from build123d import *

# Parameters (mm, degrees)
CROQUIS1_W              = 32
CROQUIS1_H              = 74.5
CROQUIS1_R              = 1.5
SALIENTE_EXTRUIR1_DEPTH = 1.5
REDONDEO1_R             = 2


with BuildPart() as part:
    # Croquis1 → Saliente-Extruir1 (new, symmetric)
    with BuildSketch(Plane.XY):
        Rectangle(CROQUIS1_W, CROQUIS1_H)
        with Locations((0, 27.25)):
            Circle(CROQUIS1_R, mode=Mode.SUBTRACT)
        with Locations((-9, 6.75)):
            Circle(CROQUIS1_R, mode=Mode.SUBTRACT)
        with Locations((9, 6.75)):
            Circle(CROQUIS1_R, mode=Mode.SUBTRACT)
    extrude(amount=SALIENTE_EXTRUIR1_DEPTH, both=True)

    # Redondeo1
    redondeo1_edges = [part.edges().sort_by_distance(p)[0] for p in [
        (-16, 37.25, 0),
        (16, 37.25, 0),
    ]]
    fillet(redondeo1_edges, radius=REDONDEO1_R)


solid = part.part
The model under review builds one solid part; all positions refer to its coordinate system, in mm. Round coordinates to 2 decimals unless told otherwise and drop trailing zeros. Order: outer loops, then holes, each group sorted by start corner. A loop starts at its lowest first (then second) coordinate and runs counter-clockwise, first axis right, second up. Notation, with made-up numbers: (-9.5, 45.25) -> (5.5, 45.25) arc R3 cw to (5.5, 49.25) -> close; hole circle Ø5 at (82, -34.5). An arc over 180 degrees is marked (long way). Write item = value, one per line. Start each with the question number.
Item 1: Consider section A-A on x = -9. Write out the cut boundary in (y, z).
Item 2: Consider section B-B on y = 27.25. Write out the cut boundary in (x, z), plus the area to 3 significant figures.
Item 3: Consider section C-C on y = 6.75. Write out the cut boundary in (x, z).
Item 4: For line 1 along Y through (x, z) = (9, -0.2); line 2 along Y through (x, z) = (0, -0.15); line 3 along X through (y, z) = (27.5, -0.45), list the stretches that pass through material, from the lowest coordinate up.
Item 5: Mouldability with a two-part tool opening along Y and no side actions: class faces 1 (the face through (0, 37.25, 0)), 2 (the face through (7.81, 5.84, -0.02)), 3 (the face through (16, -2, 0)), 4 (the face through (0, -37.25, 0)) as released by +Y, released by -Y, zero draft, split by the parting line, or undercut.
Conclusion:
q1.outline = (-37.25, -1.5) -> (5.25, -1.5) -> (5.25, 1.5) -> (-37.25, 1.5) -> close; (8.25, -1.5) -> (37.25, -1.5) -> (37.25, 1.5) -> (8.25, 1.5) -> close
q2.outline = (-16, -1.5) -> (-1.5, -1.5) -> (-1.5, 1.5) -> (-16, 1.5) -> close; (1.5, -1.5) -> (16, -1.5) -> (16, 1.5) -> (1.5, 1.5) -> close
q2.area = 87.0 mm2
q3.outline = (-16, -1.5) -> (-10.5, -1.5) -> (-10.5, 1.5) -> (-16, 1.5) -> close; (-7.5, -1.5) -> (7.5, -1.5) -> (7.5, 1.5) -> (-7.5, 1.5) -> close; (10.5, -1.5) -> (16, -1.5) -> (16, 1.5) -> (10.5, 1.5) -> close
q4.line_1 = -37.25 to 5.25, 8.25 to 37.25
q4.line_2 = -37.25 to 25.75, 28.75 to 37.25
q4.line_3 = -16 to -1.48, 1.48 to 16
q5.face_1 = released by +Y
q5.face_2 = undercut
q5.face_3 = zero draft
q5.face_4 = released by -Y
